```python
from build123d import *

# Parameters (mm, degrees)
BOSS_EXTRUDE1_DEPTH = 5
CIRPATTERN2_COUNT   = 7
BOSS_EXTRUDE3_DEPTH = 5


with BuildPart() as part:
    # Sketch1 → Boss-Extrude1 (new body)
    with BuildSketch(Plane(origin=(0, 0, 0), x_dir=(1, 0, 0), z_dir=(0, 1, 0))):
        with BuildLine():
            Line((0.5, 7.342689489), (-0.5, 7.342689489))
            ThreePointArc((-0.5, 7.342689489), (-0.952778657, 5.876485931), (-1, 4.342689489))
            Line((-1, 4.342689489), (1, 4.342689489))
            ThreePointArc((1, 4.342689489), (0.952778657, 5.876485931), (0.5, 7.342689489))
        make_face()
        with BuildLine():
            Line((0, 5.842689489), (0.9583076, 5.842689489))
            ThreePointArc((0.9583076, 5.842689489), (1.314078634, 4.820077302), (2, 3.98232997))
            Line((2, 3.98232997), (-2, 3.98232997))
            ThreePointArc((-2, 3.98232997), (-1.314078634, 4.820077302), (-0.9583076, 5.842689489))
            Line((-0.9583076, 5.842689489), (0, 5.842689489))
        make_face()
    boss_extrude1 = extrude(amount=BOSS_EXTRUDE1_DEPTH)

    # CirPattern2: Boss-Extrude1 ×7 about axis
    cirpattern2_axis = Axis((0, 0, 0), (0, 1, 0))
    for i in range(1, CIRPATTERN2_COUNT):
        add(boss_extrude1.rotate(cirpattern2_axis, i * 360 / CIRPATTERN2_COUNT))

    # Sketch1<5> → Boss-Extrude3 (add)
    with BuildSketch(Plane(origin=(0, 0, 0), x_dir=(1, 0, 0), z_dir=(0, 1, 0))):
        with BuildLine():
            ThreePointArc((4.456338407, 0), (3.792863615, 2.339473785), (2, 3.98232997))
            Line((2, 3.98232997), (-2, 3.98232997))
            ThreePointArc((-2, 3.98232997), (-2.339473785, -3.792863615), (4.456338407, 0))
        make_face()
        with BuildLine():
            ThreePointArc((1.125, 0), (0.795495129, -0.795495129), (0, -1.125))
            ThreePointArc((0, -1.125), (-1.125, 0), (0, 1.125))
            ThreePointArc((0, 1.125), (0.795495129, 0.795495129), (1.125, 0))
        make_face(mode=Mode.SUBTRACT)
    extrude(amount=BOSS_EXTRUDE3_DEPTH)


solid = part.part
```
For this review, take the finished solid that the model builds, in its own axes (mm). A direction names the side the tool comes from. Give positions to 0.01 mm unless a question says otherwise; leave off trailing zeros. Loops run counter-clockwise (first coordinate to the right, second up) from the corner with the lowest first, then second, coordinate; pieces in that order, holes last. Notation, with made-up numbers: M -16,46 L -6,46 A19 ccw -6,59 Z; hole C -36,66.5 d8. An arc over 180 degrees is marked long. One line per item, written item: value. Start each with the question number.
Q1. Draft analysis for pull direction X (two halves, no side actions). For faces 4 (the face through (5, 2.5, -0.2)), 5 (the face through (-4.597, 2.465, -2)), 6 (the face through (4.46, 2.46, 2.34)), state which applies: released by +X, released by -X, zero draft, split by the parting line, or undercut.
Q2. Machinability: for faces 1 (the face through (1.289, 2.465, -4.867)), 2 (the face through (5.647, 2.465, -3.501)), 3 (the face through (-5.66, 2.46, -3.52)), which of the approach directions +Z, -Z, +X, -X, +Y, -Y give a long, thin tool a straight path to every point of the face, cutting with its end or side? Answer none if there is none.
Q3. Add section B-B (z = -3.75). Give the boundary of the cut face in (x, y).
Q4. Add section C-C (x = -3). Give the boundary of the cut face in (y, z).
Q5. Add section A-A (z = -0.5). Give the boundary of the cut face in (x, y), and give its area (3 significant figures).
Q6. For L1, parallel to Z at x = -6, y = 3.6; L2, parallel to X at y = 3.8, z = -0.25; L3, parallel to Z at x = -4.75, y = 3.45, list the stretches that pass through material, from the lowest coordinate up.
Q7. Clearance check with flat-ended pins moving along their axes: pin 1 Ø2 at (y, z) = (3.5, -2.5) entering from -X; pin 2 Ø3 at (y, z) = (0.5, 4) entering from -X. State where each tip first meets the part, or that it passes through.
Reply:
1. face 4: released by +X
1. face 5: released by -X
1. face 6: undercut
2. face 1: -Z, +Y, -Y
2. face 2: +X, +Y, -Y
2. face 3: -X, +Y, -Y
3. outline: M -5.81,0 L 5.81,0 L 5.81,5 L -5.81,5 Z
4. outline: M 0,-4.04 L 5,-4.04 L 5,6.71 L 0,6.71 Z
5. outline: M -4.71,0 L -1.01,0 L -1.01,5 L -4.71,5 Z; M 1.01,0 L 4.71,0 L 4.71,5 L 1.01,5 Z
5. area: 37.0 mm²
6. L1: -4.25 to -4.08, 0.4 to 2.24
6. L2: -4.95 to -1.1, 1.1 to 4.95
6. L3: -4.76 to -2.32, -0.45 to 2.27
7. pin 1: x = -5.65
7. pin 2: x = -4.01
